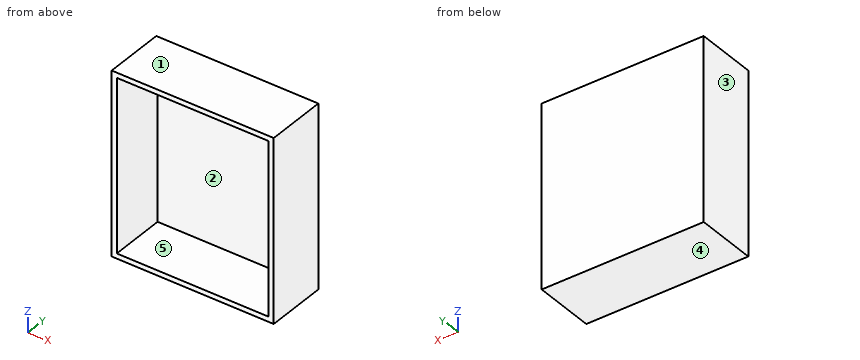
```python
from build123d import *

# Parameters (mm, degrees)
F0_W     = 203.2
F0_H     = 228.6
F0_W_2   = 190.5
F0_H_2   = 215.9
F1_DEPTH = 76.2
F2_DEPTH = 76.2
F3_DEPTH = 69.85


with BuildPart() as f1:
    # F0 (on Front) → F1 (new body)
    with BuildSketch(Plane.XZ):
        Rectangle(F0_W, F0_H)
        Rectangle(F0_W_2, F0_H_2, mode=Mode.SUBTRACT)
    extrude(amount=-F1_DEPTH)

    # F0 (on Front) → F2 (join)
    with BuildSketch(Plane.XZ):
        Rectangle(F0_W_2, F0_H_2)
    extrude(amount=-F2_DEPTH)

    # F0 (on Front) → F3 (cut)
    with BuildSketch(Plane.XZ):
        Rectangle(F0_W_2, F0_H_2)
    extrude(amount=-F3_DEPTH, mode=Mode.SUBTRACT)


solid = f1.part
```
Verification items for the finished model (mm, model axes). Face numbers are marked on the shaded views. A direction names the side the tool comes from. Coordinates: 2 decimals unless noted, no trailing zeros. Loops run counter-clockwise (first coordinate to the right, second up) from the corner with the lowest first, then second, coordinate; pieces in that order, holes last. Notation, with made-up numbers: (61.25, 24.25) -> (87.25, 24.25) arc R12 ccw to (87.25, 30.25) -> close; hole circle Ø11 at (14, -33.5). An arc over 180 degrees is marked (long way). Answer in a Markdown table with one row per item. Add a question column.
1. Section check C-C, the plane x = -28. Enter the section's corners in (y, z).
2. Depth check by flat-ended pin: P1, Ø10, axis at x = 28.5, z = -45, coming from the -Y side. Enter the tip coordinate at first touch or a pass-through.
3. Section check A-A, the plane y = 17.5. Enter the section's corners in (x, z), then the cut area to 3 significant figures.
4. Draft check along X on the marked faces 3, 4 and 5. Enter one of: +X half, -X half, draft (parallel to the pull), parting line (faces both ways), or undercut.
5. Material ranges on probe 1 along X at (y, z) = (23.5, -15); probe 2 along Z at (x, y) = (-42, 6.5); probe 3 along Y at (x, z) = (-20, -4), recorded low to high. Write a range as [from, to].
6. Access from +Z, -Z, +X, -X, +Y, -Y to the whole of each face (thin tool, end or side, straight path). Record for the marked faces 1 and 2.
7. Section check B-B, the plane z = -79. Enter the section's corners in (x, y), then the cut area to 3 significant figures.
Derived:
| question | item | result |
|---|---|---|
| 1 | outline | (0, -114.3) -> (76.2, -114.3) -> (76.2, 114.3) -> (0, 114.3) -> (0, 107.95) -> (69.85, 107.95) -> (69.85, -107.95) -> (0, -107.95) -> close |
| 2 | P1 | stops at y = 69.85 |
| 3 | outline | (-101.6, -114.3) -> (101.6, -114.3) -> (101.6, 114.3) -> (-101.6, 114.3) -> close; hole (-95.25, -107.95) -> (95.25, -107.95) -> (95.25, 107.95) -> (-95.25, 107.95) -> close |
| 3 | area | 5,320 mm² |
| 4 | face 3 | -X half |
| 4 | face 4 | draft |
| 4 | face 5 | undercut |
| 5 | probe 1 | x = [-101.6, -95.25], [95.25, 101.6] |
| 5 | probe 2 | z = [-114.3, -107.95], [107.95, 114.3] |
| 5 | probe 3 | y = [69.85, 76.2] |
| 6 | face 1 | +Z, +X, -X, +Y, -Y |
| 6 | face 2 | -Y |
| 7 | outline | (-101.6, 0) -> (-95.25, 0) -> (-95.25, 69.85) -> (95.25, 69.85) -> (95.25, 0) -> (101.6, 0) -> (101.6, 76.2) -> (-101.6, 76.2) -> close |
| 7 | area | 2,180 mm² |
